```python
from build123d import *

# Parameters (mm, degrees)
SKETCH1_W           = 40
SKETCH1_H           = 64
BOSS_EXTRUDE1_DEPTH = 3
SKETCH3_R           = 1.3
CUT_EXTRUDE2_DEPTH  = 39.209946349
SKETCH4_R           = 1.75
CUT_EXTRUDE3_DEPTH  = 39.209946349
SKETCH5_W           = 16
SKETCH5_H           = 5
SKETCH5_H_2         = 8
CUT_EXTRUDE4_DEPTH  = 39.209946349
FILLET1_R           = 2
FILLET2_R           = 4
FILLET3_R           = 1


with BuildPart() as part:
    # Sketch1 → Boss-Extrude1 (new, symmetric)
    with BuildSketch(Plane.XY):
        Rectangle(SKETCH1_W, SKETCH1_H)
    extrude(amount=BOSS_EXTRUDE1_DEPTH, both=True)

    # Sketch3 → Cut-Extrude2 (cut, through all)
    with BuildSketch(Plane.XY.offset(3)):
        with Locations((-15.2, 21)):
            Circle(SKETCH3_R)
        with Locations((15.2, 5)):
            Circle(SKETCH3_R)
        with Locations((-15.2, -5)):
            Circle(SKETCH3_R)
        with Locations((15.2, -21)):
            Circle(SKETCH3_R)
    extrude(amount=-CUT_EXTRUDE2_DEPTH, mode=Mode.SUBTRACT)

    # Sketch4 → Cut-Extrude3 (cut, through all)
    with BuildSketch(Plane.XY.offset(3)):
        with Locations((0, -28)):
            Circle(SKETCH4_R)
        with Locations(Location((0, 28, 0), (0, 0, 180))):
            Circle(SKETCH4_R)
    extrude(amount=-CUT_EXTRUDE3_DEPTH, mode=Mode.SUBTRACT)

    # Sketch5 → Cut-Extrude4 (cut, through all)
    with BuildSketch(Plane.XY.offset(3)):
        with Locations((-12, 0)):
            Rectangle(SKETCH5_W, SKETCH5_H)
        with Locations((12, 0)):
            Rectangle(SKETCH5_W, SKETCH5_H)
        with Locations((12, -28)):
            Rectangle(SKETCH5_W, SKETCH5_H_2)
        with Locations((-12, -28)):
            Rectangle(SKETCH5_W, SKETCH5_H_2)
        with Locations((12, 28)):
            Rectangle(SKETCH5_W, SKETCH5_H_2)
        with Locations((-12, 28)):
            Rectangle(SKETCH5_W, SKETCH5_H_2)
        with BuildLine():
            Line((12.5, -18), (-12.5, -18))
            ThreePointArc((-12.5, -18), (-17.5, -13), (-12.5, -8))
            Line((-12.5, -8), (12.5, -8))
            ThreePointArc((12.5, -8), (17.5, -13), (12.5, -18))
        make_face()
        with BuildLine():
            Line((12.5, 18), (-12.5, 18))
            ThreePointArc((-12.5, 18), (-17.5, 13), (-12.5, 8))
            Line((-12.5, 8), (12.5, 8))
            ThreePointArc((12.5, 8), (17.5, 13), (12.5, 18))
        make_face()
    extrude(amount=-CUT_EXTRUDE4_DEPTH, mode=Mode.SUBTRACT)

    # Fillet1
    fillet1_edges = [part.edges().sort_by_distance(p)[0] for p in [
        (4, -2.5, 0),
        (4, 2.5, 0),
        (-4, 2.5, 0),
        (-4, -2.5, 0),
    ]]
    fillet(fillet1_edges, radius=FILLET1_R)

    # Fillet2
    fillet2_edges = [part.edges().sort_by_distance(p)[0] for p in [
        (4, -32, 0),
        (-4, -32, 0),
        (-4, 32, 0),
        (4, 32, 0),
        (20, 24, 0),
        (20, 2.5, 0),
        (-20, 24, 0),
        (-20, 2.5, 0),
        (-20, -24, 0),
        (-20, -2.5, 0),
        (20, -24, 0),
        (20, -2.5, 0),
    ]]
    fillet(fillet2_edges, radius=FILLET2_R - 0.0001)  # a hair under: the kernel refuses the full size

    # Fillet3
    fillet3_edges = [part.edges().sort_by_distance(p)[0] for p in [
        (4, 24, 0),
        (4, -24, 0),
        (-4, -24, 0),
        (-4, 24, 0),
    ]]
    fillet(fillet3_edges, radius=FILLET3_R)


solid = part.part
```
CAD build for the part. Positions are in the model's coordinates, mm. A direction names the side the tool comes from. Round coordinates to 2 decimals unless told otherwise and drop trailing zeros. Write each loop counter-clockwise with the first axis right and the second up, starting at its lowest first coordinate (ties: lowest second). Pieces come first, ordered by that corner, then holes. Notation, with made-up numbers: (4.5, 28.25) -> (57.5, 28.25) arc R35 cw to (57.5, 62.25) -> close; hole circle Ø7 at (-27.5, 46.25). An arc over 180 degrees is marked (long way). Answer in a Markdown table with one row per item. Add a question column.
Item 1: Drill centre lines: line 1 (Y direction, x = 0, z = 0.05); line 2 (Y direction, x = 12.5, z = -2.1); line 3 (X direction, y = 10, z = 0.65). Where is each one in solid material? Low to high. Write a range as from..to.
Item 2: Saw through at D-D, the plane y = -13. Write the cut outline in (x, z).
Item 3: Mould opens along X. For faces 1 (the face through (-4, -27, 0)), 2 (the face through (-11, 2.5, 0)), 3 (the face through (-0.228, -26.265, 0.042)) say: pulls with the +X half, pulls with the -X half, needs draft (parallel to the pull), parting line crosses it, or undercut.
Item 4: Saw through at A-A, the plane y = -5. Write the cut outline in (x, z).
Item 5: Saw through at C-C, the plane z = -2.25. Count the separate pieces of the cut face and the enclosed holes in it, then the cut area to 3 significant figures.
Item 6: Which spindle directions (+Z, -Z, +X, -X, +Y, -Y) get a long thin tool onto all of the face, cutting with end or side? Do faces 4 (the face through (-17.5, 13.1, 0)), 5 (the face through (-2.859, -30.797, -0.042)), 6 (the face through (-4.6, -1.93, -0.04)), 7 (the face through (18.859, -3.703, -0.042)), 8 (the face through (4, 26, 0)). Say none if no direction does.
Item 7: Drop flat-ended pins along their axis: pin 1 Ø3 at (x, z) = (10, 0.5) entering from +Y; pin 2 Ø2 at (x, y) = (15.2, -21) entering from -Z; pin 3 Ø2 at (y, z) = (23, -1) entering from -X; pin 4 Ø2.5 at (y, z) = (-26, 0) entering from +X. Give the stop position or say it passes through.
Item 8: Saw through at B-B, the plane x = -15.2. Write the cut outline in (y, z), then the cut area to 3 significant figures.
Findings below:
| question | item | result |
|---|---|---|
| 1 | line 1 | y = -32..-29.75, -26.25..-18, -8..8, 18..26.25, 29.75..32 |
| 1 | line 2 | y = -24..-18, -8..-2.5, 2.5..8, 18..24 |
| 1 | line 3 | x = -20..-16.5, 16.5..20 |
| 2 | outline | (-20, -3) -> (-17.5, -3) -> (-17.5, 3) -> (-20, 3) -> close; (17.5, -3) -> (20, -3) -> (20, 3) -> (17.5, 3) -> close |
| 3 | face 1 | pulls with the -X half |
| 3 | face 2 | needs draft |
| 3 | face 3 | undercut |
| 4 | outline | (-19.71, -3) -> (-16.5, -3) -> (-16.5, 3) -> (-19.71, 3) -> close; (-13.9, -3) -> (19.71, -3) -> (19.71, 3) -> (-13.9, 3) -> close |
| 5 | separate pieces | 1 |
| 5 | enclosed holes | 8 |
| 5 | area | 1,150 mm^2 |
| 6 | face 4 | +Z, -Z |
| 6 | face 5 | +Z, -Z, -X, -Y |
| 6 | face 6 | +Z, -Z, -X |
| 6 | face 7 | +Z, -Z, +X |
| 6 | face 8 | +Z, -Z, +X, +Y |
| 7 | pin 1 | stops at y = 24 |
| 7 | pin 2 | passes through |
| 7 | pin 3 | stops at x = -19.46 |
| 7 | pin 4 | stops at x = 4.03 |
| 8 | outline | (-24, -3) -> (-17.21, -3) -> (-17.21, 3) -> (-24, 3) -> close; (-8.79, -3) -> (-6.3, -3) -> (-6.3, 3) -> (-8.79, 3) -> close; (-3.7, -3) -> (-2.5, -3) -> (-2.5, 3) -> (-3.7, 3) -> close; (2.5, -3) -> (8.79, -3) -> (8.79, 3) -> (2.5, 3) -> close; (17.21, -3) -> (19.7, -3) -> (19.7, 3) -> (17.21, 3) -> close; (22.3, -3) -> (24, -3) -> (24, 3) -> (22.3, 3) -> close |
| 8 | area | 126 mm^2 |
